from build123d import *

# Parameters (mm, degrees)
SKETCH1_W                       = 146.05
SKETCH1_H                       = 191.77
BOSS_EXTRUDE1_DEPTH             = 9.144
CUT_EXTRUDE1_DEPTH              = 6.604
CUT_EXTRUDE3_DEPTH              = 0.889
F_8_32_TAPPED_HOLE1_AT_2_COUNT  = 2
F_8_32_TAPPED_HOLE1_AT_2_PITCH  = 137.033
F_8_32_TAPPED_HOLE1_AT_3_COUNT  = 2
F_8_32_TAPPED_HOLE1_AT_3_PITCH  = 195.688868076
F_8_32_TAPPED_HOLE1_AT_4_COUNT  = 2
F_8_32_TAPPED_HOLE1_AT_4_PITCH  = 139.7
F_8_32_TAPPED_HOLE2_D           = 4.1656
F_8_32_TAPPED_HOLE2_DEPTH       = 9.0297
F_8_32_TAPPED_HOLE2_CSINK_D     = 5.334
F_8_32_TAPPED_HOLE2_CSINK_ANGLE = 90


with BuildPart() as part:
    # Sketch1 → Boss-Extrude1 (new body, symmetric)
    with BuildSketch(Plane.XY):
        Rectangle(SKETCH1_W, SKETCH1_H)
    extrude(amount=BOSS_EXTRUDE1_DEPTH, both=True)

    # Sketch4 → Cut-Extrude1 (cut)
    with BuildSketch(Plane.XY.offset(9.144)):
        with BuildLine():
            Line((-63.9953, -74.2569), (-63.9953, 74.2569))
            ThreePointArc((-63.9953, 74.2569), (-68.485428061, 76.116771939), (-70.3453, 80.6069))
            Line((-70.3453, 80.6069), (-70.3453, 83.1469))
            ThreePointArc((-70.3453, 83.1469), (-68.485428061, 87.637028061), (-63.9953, 89.4969))
            Line((-63.9953, 89.4969), (63.9953, 89.4969))
            ThreePointArc((63.9953, 89.4969), (68.485428061, 87.637028061), (70.3453, 83.1469))
            Line((70.3453, 83.1469), (70.3453, 80.6069))
            ThreePointArc((70.3453, 80.6069), (68.485428061, 76.116771939), (63.9953, 74.2569))
            Line((63.9953, 74.2569), (63.9953, -74.2569))
            ThreePointArc((63.9953, -74.2569), (68.485428061, -76.116771939), (70.3453, -80.6069))
            Line((70.3453, -80.6069), (70.3453, -83.1469))
            ThreePointArc((70.3453, -83.1469), (68.485428061, -87.637028061), (63.9953, -89.4969))
            Line((63.9953, -89.4969), (-63.9953, -89.4969))
            ThreePointArc((-63.9953, -89.4969), (-68.485428061, -87.637028061), (-70.3453, -83.1469))
            Line((-70.3453, -83.1469), (-70.3453, -80.6069))
            ThreePointArc((-70.3453, -80.6069), (-68.485428061, -76.116771939), (-63.9953, -74.2569))
        make_face()
    cut_extrude1 = extrude(amount=-CUT_EXTRUDE1_DEPTH, mode=Mode.SUBTRACT)

    # Sketch5 → Cut-Extrude3 (cut)
    with BuildSketch(Plane(origin=(0, 0, 2.54), x_dir=(-1, 0, 0), z_dir=(0, 0, -1))):
        with BuildLine():
            Line((-61.4553, 86.9569), (61.4553, 86.9569))
            ThreePointArc((61.4553, 86.9569), (67.8053, 80.6069), (61.4553, 74.2569))
            Line((61.4553, 74.2569), (61.4553, -74.2569))
            ThreePointArc((61.4553, -74.2569), (67.8053, -80.6069), (61.4553, -86.9569))
            Line((61.4553, -86.9569), (-61.4553, -86.9569))
            ThreePointArc((-61.4553, -86.9569), (-67.8053, -80.6069), (-61.4553, -74.2569))
            Line((-61.4553, -74.2569), (-61.4553, 74.2569))
            ThreePointArc((-61.4553, 74.2569), (-67.8053, 80.6069), (-61.4553, 86.9569))
        make_face()
    cut_extrude3 = extrude(amount=CUT_EXTRUDE3_DEPTH, mode=Mode.SUBTRACT)

    # Mirror1: Cut-Extrude1, Cut-Extrude3 across plane
    add(cut_extrude1.mirror(Plane.XY), mode=Mode.SUBTRACT)
    add(cut_extrude3.mirror(Plane.XY), mode=Mode.SUBTRACT)

    # Sketch8 → #8-32 Tapped Hole1 (revolve, cut)
    with BuildSketch(Plane(origin=(68.5165, 69.85, 9.144), x_dir=(0, -1, 0), z_dir=(1, 0, 0))):
        Polygon((0, 0), (0, 18.288), (2.667, 18.288), (2.0828, 17.7038), (2.0828, 0.5842), (2.667, 0), align=None)
    f_8_32_tapped_hole1 = revolve(axis=Axis((68.5165, 69.85, 15.494), (0, 0, -1)), mode=Mode.SUBTRACT)

    # #8-32 Tapped Hole1 at 2: #8-32 Tapped Hole1 ×2
    with Locations(*[(-i * F_8_32_TAPPED_HOLE1_AT_2_PITCH, 0, 0) for i in range(1, F_8_32_TAPPED_HOLE1_AT_2_COUNT)]):
        add(f_8_32_tapped_hole1, mode=Mode.SUBTRACT)

    # #8-32 Tapped Hole1 at 3: #8-32 Tapped Hole1 ×2
    with Locations(*[Vector(-0.700259557, -0.713888334, 0) * (i * F_8_32_TAPPED_HOLE1_AT_3_PITCH) for i in range(1, F_8_32_TAPPED_HOLE1_AT_3_COUNT)]):
        add(f_8_32_tapped_hole1, mode=Mode.SUBTRACT)

    # #8-32 Tapped Hole1 at 4: #8-32 Tapped Hole1 ×2
    with Locations(*[(0, -i * F_8_32_TAPPED_HOLE1_AT_4_PITCH, 0) for i in range(1, F_8_32_TAPPED_HOLE1_AT_4_COUNT)]):
        add(f_8_32_tapped_hole1, mode=Mode.SUBTRACT)

    # #8-32 Tapped Hole2
    with Locations(Plane(origin=(73.025, 0, 0), x_dir=(0, 0, -1), z_dir=(1, 0, 0))):
        with Locations((5.08, 60.325), (-5.08, -60.325), (5.08, -60.325), (-5.08, 60.325)):
            CounterSinkHole(F_8_32_TAPPED_HOLE2_D / 2, F_8_32_TAPPED_HOLE2_CSINK_D / 2, depth=F_8_32_TAPPED_HOLE2_DEPTH, counter_sink_angle=F_8_32_TAPPED_HOLE2_CSINK_ANGLE)


solid = part.part
Could you check a few things on this model? Use its own coordinates, in mm. A direction names the side the tool comes from. Give positions to 0.01 mm unless a question says otherwise; leave off trailing zeros. Order: outer loops, then holes, each group sorted by start corner. A loop starts at its lowest first (then second) coordinate and runs counter-clockwise, first axis right, second up. Notation, with made-up numbers: (43.25, 77.5) - (64.25, 77.5) arc R34 ccw to (64.25, 110.5) - close; hole circle Ø6 at (39, 1). An arc over 180 degrees is marked (long way). Return JSON: item names as keys, results as strings. Group by question number.
Q1. Suppose I cut it at A-A, the plane y = -7. Please give me the cut outline in (x, z) (3 decimals), and give its area (3 significant figures).
Q2. Please list where these lines run through material, in increasing order: line 1 along X through (y, z) = (-69.85, -1.75) (3 decimals); line 2 along X through (y, z) = (16, 7.5) (3 decimals); line 3 along Y through (x, z) = (24, 4) (3 decimals). Write a range as [from, to].
Q3. Will these pins go through, and if not, where does the flat tip stop? pin 1 Ø1.5 at (x, y) = (-39.5, -47) entering from -Z; pin 2 Ø3.5 at (y, z) = (60.325, -5.08) entering from +X; pin 3 Ø8 at (x, y) = (-18.5, 64) entering from +Z.
Q4. Suppose I cut it at B-B, the plane x = 18.5. Please give me the cut outline in (y, z) (3 decimals).
Q5. Suppose I cut it at C-C, the plane z = -5. State how many separate pieces and enclosed holes the cut face has, and give its area (3 significant figures).
Q6. Thinking about a two-plate mould opening in Z: for faces 5 (the face through (68.16, -62.36, -5.53)), 6 (the face through (-68.44, 76.07, 5.89)), 7 (the face through (66, 70, 9)), which applies, pulls with the +Z half, pulls with the -Z half, needs draft (parallel to the pull), parting line crosses it, or undercut?
Q7. Which directions (+Z, -Z, +X, -X, +Y, -Y) give clear straight access to the entire face, cutting with the end or side of a thin tool? Please do faces 1 (the face through (-73.025, -1, 0)), 2 (the face through (-67.804, 80.747, 2.102)), 3 (the face through (-67.804, 80.747, -2.102)), 4 (the face through (68.2, 58.3, 4.6)).
Resolved:
{
 "1": {"outline": "(-73.025, -9.144) - (-63.995, -9.144) - (-63.995, -2.54) - (-61.455, -2.54) - (-61.455, -1.651) - (61.455, -1.651) - (61.455, -2.54) - (63.995, -2.54) - (63.995, -9.144) - (73.025, -9.144) - (73.025, 9.144) - (63.995, 9.144) - (63.995, 2.54) - (61.455, 2.54) - (61.455, 1.651) - (-61.455, 1.651) - (-61.455, 2.54) - (-63.995, 2.54) - (-63.995, 9.144) - (-73.025, 9.144) - close", "area": "762 mm2"},
 "2": {"line 1": "x = [-73.025, -70.599], [-66.434, -61.455], [61.455, 66.434], [70.599, 73.025]", "line 2": "x = [-73.025, -63.995], [63.995, 73.025]", "line 3": "y = [-95.885, -89.497], [89.497, 95.885]"},
 "3": {"pin 1": "stops at z = -1.65", "pin 2": "stops at x = -64", "pin 3": "stops at z = 1.65"},
 "4": {"outline": "(-95.885, -9.144) - (-89.497, -9.144) - (-89.497, -2.54) - (-86.957, -2.54) - (-86.957, -1.651) - (86.957, -1.651) - (86.957, -2.54) - (89.497, -2.54) - (89.497, -9.144) - (95.885, -9.144) - (95.885, 9.144) - (89.497, 9.144) - (89.497, 2.54) - (86.957, 2.54) - (86.957, 1.651) - (-86.957, 1.651) - (-86.957, 2.54) - (-89.497, 2.54) - (-89.497, 9.144) - (-95.885, 9.144) - close"},
 "5": {"separate pieces": "2", "enclosed holes": "4", "area": "4,650 mm2"},
 "6": {"face 5": "undercut", "face 6": "needs draft", "face 7": "pulls with the +Z half"},
 "7": {"face 1": "+Z, -Z, -X, +Y, -Y", "face 2": "+Z", "face 3": "-Z", "face 4": "+X"}
}
